Autodesk Inventor part; units mm, degrees
ref_plane "Arbeitsebene1" through (0, 0, 0) normal (0, 0, 1) x (1, 0, 0)
ref_plane "YZ Plane" through (0, 0, 0) normal (1, 0, 0) x (0, 1, 0)
ref_plane "XZ Plane" through (0, 0, 0) normal (0, 1, 0) x (-1, 0, 0)
sketch "Skizze1" plane through (0, 0, 0) normal (0, 0, 1) x (1, 0, 0)
  point P0 (0, 0)
ref_plane "Arbeitsebene1" through (0, 0, 0) normal (0, 0, 1) x (1, 0, 0)
sketch "Skizze2" plane through (0, 0, 0) normal (0, 0, 1) x (1, 0, 0)
  line L0 (-10, -0.5) -> (-12, -0.5)
  line L1 (-12, -0.5) -> (-12, -23.5)
  arc A0 (-12, -23.5) -> (-10, -25.5) centre (-10, -23.5) ccw
  line L2 (-10, -25.5) -> (-9.8284, -25.5)
  arc A1 (-8.4142, -26.0858) -> (-9.8284, -25.5) centre (-9.8284, -27.5) ccw
  line L3 (0.4142, -34.9142) -> (-8.4142, -26.0858)
  arc A2 (1, -36.3284) -> (0.4142, -34.9142) centre (-1, -36.3284) ccw
  line L4 (1, -36.3284) -> (1, -46.5)
  arc A3 (1, -46.5) -> (3, -48.5) centre (3, -46.5) ccw
  line L5 (3, -48.5) -> (10, -48.5)
  arc A4 (10, -48.5) -> (12, -46.5) centre (10, -46.5) ccw
  line L6 (12, -46.5) -> (12, 31.5)
  line L7 (11, 32.5) -> (10, 32.5)
  line L8 (10, 32.5) -> (10, -46.5)
  line L9 (10, -46.5) -> (3, -46.5)
  line L10 (3, -46.5) -> (3, -23.5)
  line L11 (3, -23.5) -> (-10, -23.5)
  line L12 (-10, -23.5) -> (-10, -0.5)
  arc A5 (1, 48.5) -> (0, 47.5) centre (1, 47.5) ccw
  line L13 (0, 47.5) -> (0, 32.5)
  line L14 (0, 32.5) -> (5, 32.5)
  line L15 (5, 32.5) -> (5, 47.5)
  arc A6 (5, 47.5) -> (4, 48.5) centre (4, 47.5) ccw
  line L16 (4, 48.5) -> (1, 48.5)
  line L17 (-12, 12.5) -> (-10, 12.5)
  line L18 (-10, 12.5) -> (-10, 47.5)
  arc A7 (-10, 47.5) -> (-12, 47.5) centre (-11, 47.5) ccw
  line L19 (-12, 47.5) -> (-12, 12.5)
  line L20 (-10, 12.5) -> (-10, -0.5)
  line L21 (-12, 12.5) -> (-10, 12.5)
  line L22 (-12, -0.5) -> (-12, 12.5)
  line L23 (-10, -0.5) -> (-12, -0.5)
  arc A8 (12, 31.5) -> (11, 32.5) centre (11, 31.5) ccw
  point P0 (0, 0)
extrude "Extrusion1" add sketch "Skizze2" along normal blind 9
sketch "Skizze3" plane through (0, 0, 9) normal (0, 0, 1) x (1, 0, 0)
  line L0 (-12, 47.5) -> (-12, -23.5)
  arc A0 (-12, -23.5) -> (-10, -25.5) centre (-10, -23.5) ccw
  line L1 (-10, -25.5) -> (-9.8284, -25.5)
  arc A1 (-8.4142, -26.0858) -> (-9.8284, -25.5) centre (-9.8284, -27.5) ccw
  line L2 (-8.4142, -26.0858) -> (0.4142, -34.9142)
  arc A2 (1, -36.3284) -> (0.4142, -34.9142) centre (-1, -36.3284) ccw
  line L3 (1, -36.3284) -> (1, -46.5)
  arc A3 (1, -46.5) -> (3, -48.5) centre (3, -46.5) ccw
  line L4 (3, -48.5) -> (10, -48.5)
  arc A4 (10, -48.5) -> (12, -46.5) centre (10, -46.5) ccw
  line L5 (12, -46.5) -> (12, 31.5)
  line L6 (11, 32.5) -> (10, 32.5)
  line L7 (10, 32.5) -> (10, -46.5)
  line L8 (10, -46.5) -> (3, -46.5)
  line L9 (3, -46.5) -> (3, -23.5)
  line L10 (3, -23.5) -> (-10, -23.5)
  line L11 (-10, -23.5) -> (-10, 47.5)
  arc A5 (-10, 47.5) -> (-12, 47.5) centre (-11, 47.5) ccw
  line L12 (0, 32.5) -> (5, 32.5)
  line L13 (5, 32.5) -> (5, 47.5)
  arc A6 (5, 47.5) -> (4, 48.5) centre (4, 47.5) ccw
  line L14 (4, 48.5) -> (1, 48.5)
  arc A7 (1, 48.5) -> (0, 47.5) centre (1, 47.5) ccw
  line L15 (0, 47.5) -> (0, 32.5)
  line L16 (10, 32.5) -> (5, 32.5)
  line L17 (-11, 48.5) -> (4, 48.5)
  arc A8 (12, 31.5) -> (11, 32.5) centre (11, 31.5) ccw
  point P0 (0, 0)
extrude "Extrusion2" add sketch "Skizze3" along normal blind 2
sketch "Skizze5" plane through (-10, -23.5, 0) normal (1, 0, 0) x (0, 0, -1)
  line L0 (0, 0) -> (0, 71)
  line L1 (0, 71) -> (-9, 71)
  line L2 (-9, 0) -> (-9, 71)
  line L3 (0, 0) -> (-9, 0)
  line L4 (-9, 0) -> (-9, 71)
  line L5 (-9, 0) -> (-4, 0)
  line L6 (-4, 0) -> (-4, 5)
  line L7 (-4, 5) -> (-9, 5)
  line L8 (-9, 5) -> (-9, 0)
  point P0 (0, 23.5)
  point P1 (-9, 5)
  dimension "d4" = 5
  dimension "d5" = 5
extrude "Extrusion3" add sketch "Skizze5" along normal blind 2.5 contours L3 L2 L7 L6
sketch "Skizze6" plane through (-7.5, -23.5, 0) normal (1, 0, 0) x (0, 0, -1)
  line L0 (-4, 0) -> (-4, 5)
  line L1 (-4, 0) -> (-9, 0)
  line L2 (-4, 5) -> (-9, 5)
  line L3 (-9, 5) -> (-9, 0)
  line L4 (-9, 0) -> (-4, 0)
  line L5 (-4, 0) -> (-4, 5)
  point P0 (0, 23.5)
extrude "Extrusion4" cut sketch "Skizze6" against normal blind 1
sketch "Skizze7" plane through (0, 0, 0) normal (0, 0, -1) x (-1, 0, 0)
  line L0 (0, 32.5) -> (-5, 32.5)
  line L1 (0, 32.5) -> (-3.8, 32.5)
  line L2 (-3.8, 32.5) -> (-3.8, 34.5)
  line L3 (-3.8, 34.5) -> (0, 34.5)
  line L4 (0, 34.5) -> (0, 32.5)
  point P0 (0, 0)
  dimension "d10" = 2
  dimension "d11" = 3.8
extrude "Extrusion5" cut sketch "Skizze7" against normal up to surface (9 mm away)
sketch "Skizze8" plane through (0, 0, 11) normal (0, 0, 1) x (1, 0, 0)
  line L0 (3.8, 32.5) -> (5, 32.5)
  line L1 (12, -46.5) -> (12, 31.5)
  line L2 (5, 32.5) -> (12, 32.5)
  line L3 (12, 32.5) -> (12, 29.5)
  line L4 (12, 29.5) -> (5, 29.5)
  line L5 (5, 29.5) -> (5, 32.5)
  point P0 (0, 0)
  dimension "d14" = 3
extrude "Extrusion6" cut sketch "Skizze8" against normal through all
sketch "Skizze9" plane through (5, 32.5, 0) normal (0, -1, 0) x (1, 0, 0)
  line L0 (-1.2, 0) -> (-1.2, 9)
  line L1 (0, 0) -> (0, 11)
  line L2 (-1.2, 0) -> (0, 0)
  line L3 (0, 0) -> (0, 9)
  line L4 (0, 9) -> (-1.2, 9)
  line L5 (-1.2, 9) -> (-1.2, 0)
  point P0 (-5, 0)
  dimension "d17" = 9
extrude "Extrusion7" add sketch "Skizze9" along normal blind 3
sketch "Skizze10" plane through (-12, -23.5, 0) normal (-1, 0, 0) x (0, 0, 1)
  line L0 (0, 0) -> (0, 71)
  line L1 (0, 23.8) -> (1.5, 23.8)
  line L2 (1.5, 23.8) -> (1.5, 38.5)
  line L3 (1.5, 38.5) -> (0, 38.5)
  line L4 (0, 38.5) -> (0, 23.8)
  line L5 (0, 71) -> (11, 71)
  point P0 (0, 23.5)
  point P1 (0, 38.5)
  dimension "d20" = 1.5
  dimension "d21" = 14.7
  dimension "d57" = 23.8
extrude "Extrusion8" cut sketch "Skizze10" against normal up to surface (22 mm away)
sketch "Skizze11" plane through (0, 0, 9) normal (0, 0, -1) x (-1, 0, 0)
  line L0 (-4, 48.5) -> (11, 48.5)
  line L1 (7.2, 48.5) -> (2.2, 48.5)
  line L2 (2.2, 48.5) -> (2.2, 43.6)
  line L3 (2.2, 43.6) -> (7.2, 43.6)
  line L4 (7.2, 43.6) -> (7.2, 48.5)
  line L5 (12, 47.5) -> (12, 15)
  point P0 (0, 0)
  point P1 (2.2, 48.5)
  dimension "d25" = 4.9
  dimension "d26" = 5
  dimension "d27" = 4.8
extrude "Extrusion9" cut sketch "Skizze11" against normal blind 3
sketch "Skizze12" plane through (0, 0, 0) normal (0, 0, -1) x (-1, 0, 0)
  line L0 (-3, -23.5) -> (10, -23.5)
  line L1 (-3, -46.5) -> (-3, -23.5)
  point P0 (0, 0)
  point P1 (1, -27.5)
  dimension "d30" = 4
  dimension "d31" = 4
hole "Bohrung1" at (-1, -27.5, 0) direction (0, 0, 1) diameter 2 end through all
sketch "Skizze13" plane through (0, 0, 0) normal (0, 0, -1) x (-1, 0, 0)
  line L0 (-5, 29.5) -> (-5, 47.5)
  line L1 (-4, 48.5) -> (-1, 48.5)
  point P0 (0, 0)
  point P1 (-2.5, 41.5)
  dimension "d39" = 2.5
  dimension "d40" = 7
hole "Bohrung2" at (2.5, 41.5, 0) direction (0, 0, 1) diameter 2 end through all
sketch "Skizze14" plane through (-8.5, -23.5, 0) normal (1, 0, 0) x (0, 0, -1)
  line L0 (-9, 5) -> (-4, 5)
  line L1 (-4, 5) -> (-4, 0)
  point P0 (0, 23.5)
  point P1 (-6.5, 2.5)
  dimension "d48" = 2.5
  dimension "d49" = 2.5
hole "Bohrung3" at (-8.5, -21, 6.5) direction (-1, 0, 0) diameter 2.5 end through all
sketch "Skizze16" plane through (0, 0, 0) normal (0, 0, -1) x (-1, 0, 0)
  line L0 (-5, 29.5) -> (-10, 29.5)
  line L1 (-10, 29.5) -> (-10.5, 29.5)
  line L2 (-10.5, 29.5) -> (-10.5, 19.5)
  line L3 (-10.5, 19.5) -> (-10, 19.5)
  line L4 (-10, 19.5) -> (-10, 29.5)
  point P0 (0, 0)
  dimension "d63" = 0.5
  dimension "d64" = 10
extrude "Extrusion11" cut sketch "Skizze16" against normal up to surface (9 mm away)
properties part number "Case" material "Holz (Eiche)"
Geometry check sheet. Reference: the model listing, model coordinates, mm. A direction names the side the tool comes from. Round coordinates to 2 decimals unless told otherwise and drop trailing zeros. Write each loop counter-clockwise with the first axis right and the second up, starting at its lowest first coordinate (ties: lowest second). Pieces come first, ordered by that corner, then holes. Notation, with made-up numbers: (72, 88) - (102, 88) arc R5 ccw to (102, 96) - close; hole circle Ø5 at (35, 50). An arc over 180 degrees is marked (long way). Write each question's results on one line, items separated by ' | '.
(1) Depth check by flat-ended pin: pin 1 Ø2 at (x, y) = (-6, -22) entering from -Z; pin 2 Ø3.5 at (x, z) = (6.5, 5) entering from +Y; pin 3 Ø2 at (y, z) = (45, 10) entering from +X. Enter the tip coordinate at first touch or a pass-through.
Computed:
pin 1: stops at z = 9 | pin 2: stops at y = 48.16 | pin 3: stops at x = 5
(2) Sectioned sample at B-B, the plane z = 2.75. Count the separate pieces of the cut face and the enclosed holes in it, plus the area to 3 significant figures.
Computed:
separate pieces: 2 | enclosed holes: 2 | area: 501 mm^2
(3) Sectioned sample at A-A, the plane x = -1. Enter the section's corners in (y, z).
Computed:
outline: (-33.5, 0) - (-28.5, 0) - (-28.5, 11) - (-33.5, 11) - close; (-26.5, 0) - (-23.5, 0) - (-23.5, 9) - (48.5, 9) - (48.5, 11) - (-26.5, 11) - close
(4) Thickness scan on probe 1 along X at (y, z) = (20, 2); probe 2 along X at (y, z) = (1.5, 2); probe 3 along X at (y, z) = (-27.5, 6.25). Record the ranges inside material, lowest first. Write a range as from..to.
Computed:
probe 1: x = -12..-10, 10.5..12 | probe 2: x = -12..-10, 10..12 | probe 3: x = -7..-2, 0..3, 10..12
(5) Set-up check for faces 1 (the face through (-5, 43.6, 10)), 2 (the face through (5, 39, 5)), 3 (the face through (-11, 48.5, 5.4)): record each of +Z, -Z, +X, -X, +Y, -Y from which the full face is reachable in a straight line by a thin tool's end or side.
Computed:
face 1: +Z, -Z, +Y | face 2: +Z, -Z, +X, +Y | face 3: -Z, +Y
(6) Sectioned sample at C-C, the plane y = -27.5. Enter the section's corners in (x, z), plus the area to 3 significant figures.
Computed:
outline: (-7, 0) - (-2, 0) - (-2, 11) - (-7, 11) - close; (0, 0) - (3, 0) - (3, 9) - (10, 9) - (10, 0) - (12, 0) - (12, 11) - (0, 11) - close | area: 124 mm^2
(7) Draft check along Z on faces 4 (the face through (-10, 12, 4)), 5 (the face through (-11, 8, 1.5)), 6 (the face through (0, 1, 11)). Enter one of: pulls with the +Z half, pulls with the -Z half, needs draft (parallel to the pull), parting line crosses it, or undercut.
Computed:
face 4: needs draft | face 5: pulls with the -Z half | face 6: pulls with the +Z half
